from build123d import *

# Parameters (mm, degrees)
ESQUISSE1_R                                   = 5.5
ESQUISSE1_R_2                                 = 4.5
BOSS_EXTRU_1_DEPTH                            = 10
ESQUISSE3_R                                   = 8.5
ESQUISSE3_R_2                                 = 5
BOSS_EXTRU_3_DEPTH                            = 7
ESQUISSE4_R                                   = 9
ESQUISSE4_R_2                                 = 5
BOSS_EXTRU_4_DEPTH                            = 2
ESQUISSE7_R                                   = 6
ESQUISSE7_R_2                                 = 5
BOSS_EXTRU_7_DEPTH                            = 11
ESQUISSE8_R                                   = 9
ESQUISSE8_R_2                                 = 5
BOSS_EXTRU_8_DEPTH                            = 2
ESQUISSE15_R                                  = 8.5
ESQUISSE15_R_2                                = 5
BOSS_EXTRU_9_DEPTH                            = 7
ESQUISSE16_R                                  = 5
BOSS_EXTRU_10_DEPTH                           = 5
TROU_POUR_TARAUDAGE_POUR_TROU_TARAUD_M2_D     = 1.6
TROU_POUR_TARAUDAGE_POUR_TROU_TARAUD_M2_DEPTH = 9
ENL_V_MAT_EXTRU_1_DEPTH                       = 5
D_GAGEMENT_M21_D                              = 2.2
CONG_1_R                                      = 0.5


with BuildPart() as part:
    # Esquisse1 → Boss.-Extru.1 (new body)
    with BuildSketch(Plane.XY):
        Circle(ESQUISSE1_R)
        Circle(ESQUISSE1_R_2, mode=Mode.SUBTRACT)
    extrude(amount=BOSS_EXTRU_1_DEPTH)

    # Esquisse3 → Boss.-Extru.3 (add)
    with BuildSketch(Plane.XY.offset(10)):
        Circle(ESQUISSE3_R)
        Circle(ESQUISSE3_R_2, mode=Mode.SUBTRACT)
    extrude(amount=BOSS_EXTRU_3_DEPTH)

    # Esquisse4 → Boss.-Extru.4 (add)
    with BuildSketch(Plane.XY.offset(17)):
        Circle(ESQUISSE4_R)
        Circle(ESQUISSE4_R_2, mode=Mode.SUBTRACT)
    extrude(amount=BOSS_EXTRU_4_DEPTH)

    # Esquisse7 → Boss.-Extru.7 (add)
    with BuildSketch(Plane.XY.offset(19)):
        Circle(ESQUISSE7_R)
        Circle(ESQUISSE7_R_2, mode=Mode.SUBTRACT)
    extrude(amount=BOSS_EXTRU_7_DEPTH)

    # Esquisse8 → Boss.-Extru.8 (add)
    with BuildSketch(Plane.XY.offset(30)):
        Circle(ESQUISSE8_R)
        Circle(ESQUISSE8_R_2, mode=Mode.SUBTRACT)
    extrude(amount=BOSS_EXTRU_8_DEPTH)

    # Esquisse15 → Boss.-Extru.9 (add)
    with BuildSketch(Plane.XY.offset(32)):
        Circle(ESQUISSE15_R)
        Circle(ESQUISSE15_R_2, mode=Mode.SUBTRACT)
    extrude(amount=BOSS_EXTRU_9_DEPTH)

    # Esquisse16 → Boss.-Extru.10 (add)
    with BuildSketch(Plane.XY.offset(39)):
        with BuildLine():
            Line((-5.291502622, 1.5), (-8.366600265, 1.5))
            ThreePointArc((-8.366600265, 1.5), (-8.5, 0), (-8.366600265, -1.5))
            Line((-8.366600265, -1.5), (-5.291502622, -1.5))
            ThreePointArc((-5.291502622, -1.5), (0, -5.5), (5.291502622, -1.5))
            Line((5.291502622, -1.5), (8.366600265, -1.5))
            ThreePointArc((8.366600265, -1.5), (8.5, 0), (8.366600265, 1.5))
            Line((8.366600265, 1.5), (5.291502622, 1.5))
            ThreePointArc((5.291502622, 1.5), (0, 5.5), (-5.291502622, 1.5))
        make_face()
        Circle(ESQUISSE16_R, mode=Mode.SUBTRACT)
    extrude(amount=BOSS_EXTRU_10_DEPTH)

    # Trou pour taraudage pour trou taraudé M21
    with Locations(Plane(origin=(0, 0, 10), x_dir=(-1, 0, 0), z_dir=(0, 0, -1))):
        with Locations((-7, 0), (-4.949747468, 4.949747468), (0, 7), (4.949747468, 4.949747468), (7, 0), (4.949747468, -4.949747468), (0, -7), (-4.949747468, -4.949747468), (0, 0)):
            Hole(TROU_POUR_TARAUDAGE_POUR_TROU_TARAUD_M2_D / 2, depth=TROU_POUR_TARAUDAGE_POUR_TROU_TARAUD_M2_DEPTH)

    # Esquisse17 → Enlèv. mat.-Extru.1 (cut)
    with BuildSketch(Plane.XY.offset(44)):
        with BuildLine():
            Line((-4.974937186, 0.5), (-8.485281374, 0.5))
            ThreePointArc((-8.485281374, 0.5), (-8.5, 0), (-8.485281374, -0.5))
            Line((-8.485281374, -0.5), (-4.974937186, -0.5))
            ThreePointArc((-4.974937186, -0.5), (-5, 0), (-4.974937186, 0.5))
        make_face()
        with BuildLine():
            Line((8.485281374, 0.5), (4.974937186, 0.5))
            ThreePointArc((4.974937186, 0.5), (5, 0), (4.974937186, -0.5))
            Line((4.974937186, -0.5), (8.485281374, -0.5))
            ThreePointArc((8.485281374, -0.5), (8.5, 0), (8.485281374, 0.5))
        make_face()
    extrude(amount=-ENL_V_MAT_EXTRU_1_DEPTH, mode=Mode.SUBTRACT)

    # Dégagement M21 (through all)
    with Locations(Plane(origin=(0, 1.5, 0), x_dir=(1, 0, 0), z_dir=(0, 1, 0))):
        with Locations((7.191502622, -42), (-7.191502622, -42)):
            Hole(D_GAGEMENT_M21_D / 2)

    # Congé1
    cong_1_edges = [part.edges().sort_by_distance(p)[0] for p in [
        (5.291502622, 1.5, 41.5),
        (-5.291502622, 1.5, 41.5),
        (-5.291502622, -1.5, 41.5),
        (5.291502622, -1.5, 41.5),
    ]]
    fillet(cong_1_edges, radius=CONG_1_R)


solid = part.part
Input: part model. Units: mm. Frame: model coordinates. A direction names the side the tool comes from. Give positions to 0.01 mm unless a question says otherwise; leave off trailing zeros. Loops run counter-clockwise (first coordinate to the right, second up) from the corner with the lowest first, then second, coordinate; pieces in that order, holes last. Notation, with made-up numbers: M -30,71.5 L -4,71.5 A17 cw -4,89.5 Z; hole C -2,30 d6. An arc over 180 degrees is marked long. Use CSV: the item, a comma, the result in double quotes.
(1) Set-up query: faces 1 (the face through (2, -6, 30)), 2 (the face through (-0.1, -5.5, 41.5)), 3 (the face through (8, -3.3, 32)), 4 (the face through (-7, 0, 39)). Return all of +Z, -Z, +X, -X, +Y, -Y with unobstructed straight access to the full face (end or side cutting, diameter ignored); none if empty.
Outcome:
face 1,"none"
face 2,"+Z, -Y"
face 3,"+Z"
face 4,"+Z, +X, -X"
(2) Pull-direction query (Z, two-part tool) for faces 5 (the face through (7, 0, 39)), 6 (the face through (6, 1.5, 41)), 7 (the face through (-6.38, 0.99, 41.26)), 8 (the face through (-5, 0, 0)); classes: pulls with the +Z half, pulls with the -Z half, needs draft (parallel to the pull), parting line crosses it, or undercut.
Outcome:
face 5,"pulls with the +Z half"
face 6,"needs draft"
face 7,"undercut"
face 8,"pulls with the -Z half"
(3) Section B-B, the plane z = 42. Count the separate pieces of the cut face and the enclosed holes in it, plus the area to 3 significant figures.
Outcome:
separate pieces,"6"
enclosed holes,"0"
area,"18.9 mm²"
(4) Section C-C, the plane z = 27. Return loops of the section in (x, y).
Outcome:
outline,"C 0,0 d12; hole C 0,0 d10"
(5) Section A-A, the plane y = -7. Return loops of the section in (x, z).
Outcome:
outline,"M -5.66,17 L -4.82,17 L -4.82,10 L -0.8,10 L -0.8,19 L -5.66,19 Z; M -5.66,30 L 5.66,30 L 5.66,32 L 4.82,32 L 4.82,39 L -4.82,39 L -4.82,32 L -5.66,32 Z; M 0.8,10 L 4.82,10 L 4.82,17 L 5.66,17 L 5.66,19 L 0.8,19 Z"
(6) Material intervals for L1, parallel to Z at x = 7.25, y = -1; L2, parallel to Y at x = 0, z = 13.75; L3, parallel to Z at x = -4.75, y = 6.25, sorted ascending. Write a range as [from, to].
Outcome:
L1,"z = [10, 19], [30, 40.9], [43.1, 44]"
L2,"y = [-8.5, -7.8], [-6.2, -5], [5, 6.2], [7.8, 8.5]"
L3,"z = [10, 19], [30, 39]"
(7) Pin query (flat end, axial travel): P1, Ø0.8, axis at x = -7.5, z = 42, coming from the +Y side; P2, Ø2, axis at x = -4.95, y = -4.95, coming from the +Z side; P3, Ø3.5, axis at x = 7.19, z = 42, coming from the -Y side; P4, Ø6, axis at y = -3, z = 5.5, coming from the +X side. Return the tip coordinate at first contact, or that it passes through.
Outcome:
P1,"passes through"
P2,"stops at z = 39"
P3,"stops at y = -1.55"
P4,"stops at x = 5.5"
